Geometry check sheet. Reference: the model listing, model coordinates, mm. Face numbers are marked on the shaded views. Give positions to 0.01 mm unless a question says otherwise; leave off trailing zeros. Loops run counter-clockwise (first coordinate to the right, second up) from the corner with the lowest first, then second, coordinate; pieces in that order, holes last. Notation, with made-up numbers: (89, -32) -> (148, -32) arc R16 cw to (148, -4) -> close; hole circle Ø7 at (-33.75, 43). An arc over 180 degrees is marked (long way). One line per question, with ' | ' between items.
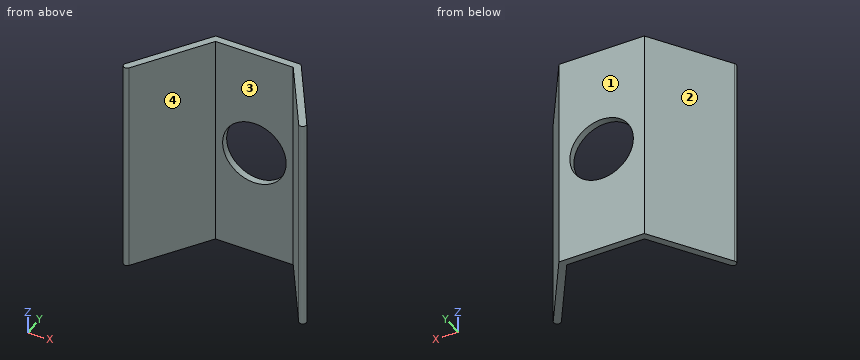
from build123d import *

# Parameters (mm, degrees)
BOSS_EXTRUDE1_DEPTH  = 7.5
M4_CLEARANCE_HOLE1_D = 4.5


with BuildPart() as part:
    # Sketch1 → Boss-Extrude1 (new, symmetric)
    with BuildSketch(Plane.XY):
        with BuildLine():
            Line((-2.75, 0), (2.75, 0))
            Line((2.75, 0), (6, -5.04356025))
            ThreePointArc((6, -5.04356025), (6.34556501, -5.118291928), (6.420296688, -4.772726917))
            Line((6.420296688, -4.772726917), (3.022624878, 0.5))
            Line((3.022624878, 0.5), (-3.022624878, 0.5))
            Line((-3.022624878, 0.5), (-6.420296688, -4.772726917))
            ThreePointArc((-6.420296688, -4.772726917), (-6.34556501, -5.118291928), (-6, -5.04356025))
            Line((-6, -5.04356025), (-2.75, 0))
        make_face()
    extrude(amount=BOSS_EXTRUDE1_DEPTH, both=True)

    # M4 Clearance Hole1 (through all)
    with Locations(Plane(origin=(0, 0.5, 0), x_dir=(1, 0, 0), z_dir=(0, 1, 0))):
        with Locations((0, 0)):
            Hole(M4_CLEARANCE_HOLE1_D / 2)


solid = part.part
Item 1: Sectioned sample at B-B (z = 0). Record the cut outline in (x, y).
Result:
outline: (-6.42, -4.77) arc R0.25 ccw to (-6, -5.04) -> (-2.75, 0) -> (-2.25, 0) -> (-2.25, 0.5) -> (-3.02, 0.5) -> close; (2.25, 0) -> (2.75, 0) -> (6, -5.04) arc R0.25 ccw to (6.42, -4.77) -> (3.02, 0.5) -> (2.25, 0.5) -> close
Item 2: Scan lines: probe 1 along Z at (x, y) = (0, 0.25); probe 2 along Y at (x, z) = (1, -5.5); probe 3 along X at (y, z) = (-3.55, -1). Record each from-to range of solid material in increasing order.
Result:
probe 1: -7.5 to -2.25, 2.25 to 7.5 | probe 2: 0 to 0.5 | probe 3: -5.63 to -5.04, 5.04 to 5.63
Item 3: Depth check by flat-ended pin: pin 1 Ø3 at (x, z) = (-1, 2.5) entering from -Y; pin 2 Ø5 at (x, z) = (-0.5, -1) entering from -Y; pin 3 Ø1 at (x, z) = (4, -5) entering from +Y. Enter the tip coordinate at first touch or a pass-through.
Result:
pin 1: y = 0 | pin 2: y = -0.39 | pin 3: y = -0.24
Item 4: Sectioned sample at A-A (x = 0). Record the cut outline in (y, z), plus the area to 3 significant figures.
Result:
outline: (0, -7.5) -> (0.5, -7.5) -> (0.5, -2.25) -> (0, -2.25) -> close; (0, 2.25) -> (0.5, 2.25) -> (0.5, 7.5) -> (0, 7.5) -> close | area: 5.25 mm2
Item 5: Sectioned sample at D-D (z = -4.5). Record the cut outline in (x, y), plus the area to 3 significant figures.
Result:
outline: (-6.42, -4.77) arc R0.25 ccw to (-6, -5.04) -> (-2.75, 0) -> (2.75, 0) -> (6, -5.04) arc R0.25 ccw to (6.42, -4.77) -> (3.02, 0.5) -> (-3.02, 0.5) -> close | area: 9.22 mm2
Item 6: Release check for a two-part mould opening along X. For the marked faces 1, 2, 3 and 4 record: pulls with the +X half, pulls with the -X half, needs draft (parallel to the pull), parting line crosses it, or undercut.
Result:
face 1: needs draft | face 2: pulls with the -X half | face 3: undercut | face 4: undercut
Item 7: Sectioned sample at C-C (y = -3.7). Record the cut outline in (x, z), plus the area to 3 significant figures.
Result:
outline: (-5.73, -7.5) -> (-5.13, -7.5) -> (-5.13, 7.5) -> (-5.73, 7.5) -> close; (5.13, -7.5) -> (5.73, -7.5) -> (5.73, 7.5) -> (5.13, 7.5) -> close | area: 17.8 mm2
